Could you check a few things on this model? Use its own coordinates, in mm. Give positions to 0.01 mm unless a question says otherwise; leave off trailing zeros. Write each loop counter-clockwise with the first axis right and the second up, starting at its lowest first coordinate (ties: lowest second). Pieces come first, ordered by that corner, then holes. Notation, with made-up numbers: (16, 78) - (51, 78) arc R26 cw to (51, 101) - close; hole circle Ø1 at (30.25, 62.25). An arc over 180 degrees is marked (long way). Use one line per item in the form item = value.
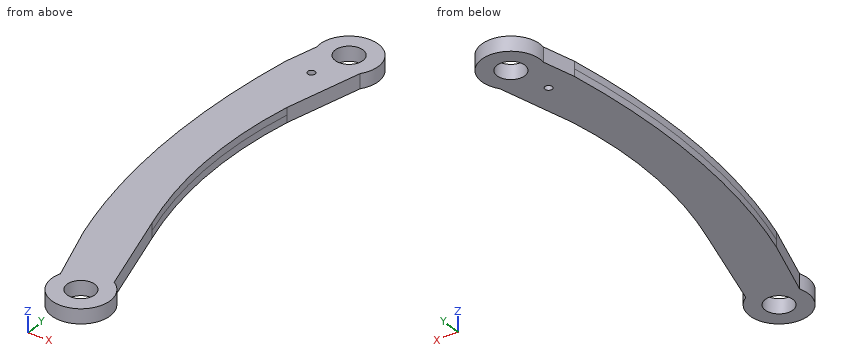
```python
from build123d import *

# Parameters (mm, degrees)
SKETCH1_R           = 1
SKETCH1_W           = 7.92
SKETCH1_H           = 7.92
SKETCH1_R_2         = 3.8
BOSS_EXTRUDE1_DEPTH = 2
SKETCH2_R           = 8
SKETCH2_W           = 7.92
SKETCH2_H           = 7.92
BOSS_EXTRUDE2_DEPTH = 2


with BuildPart() as part:
    # Sketch1 → Boss-Extrude1 (new body, symmetric)
    with BuildSketch(Plane.XY):
        with BuildLine():
            Line((-5.004193268, -11.768083729), (1.264827755, 12.086469882))
            ThreePointArc((1.264827755, 12.086469882), (-3.646245645, 20.982534185), (-12.767631248, 16.503814873))
            Line((-12.767631248, 16.503814873), (-16.10900409, 3.908669428))
            add(Edge.make_bspline(
                [(-16.10900409, 3.908669428), (-19.377716834, -15.242508961), (-20.646085271, -43.801923377), (-15.357286602, -71.564124193), (-13.027019985, -79.992281382)],
                knots=[0, 0, 0, 0, 0.615830564, 0.891753854, 0.891753854, 0.891753854, 0.891753854], degree=3))
            Line((-13.027019985, -79.992281382), (-5.967709179, -101.821397306))
            ThreePointArc((-5.967709179, -101.821397306), (-2.543292548, -94.302394888), (5.340555406, -96.773622937))
            Line((5.340555406, -96.773622937), (-2.58265982, -68.335822015))
            add(Edge.make_bspline(
                [(-2.58265982, -68.335822015), (-10.677441901, -40.31981723), (-5.004193268, -11.768083729)],
                knots=[0, 0, 0, 1, 1, 1], degree=2))
        make_face()
        with Locations((-8.672039016, 3.248347704)):
            Circle(SKETCH1_R, mode=Mode.SUBTRACT)
        with Locations((-5.857463234, 13.958219751)):
            Rectangle(SKETCH1_W, SKETCH1_H, mode=Mode.SUBTRACT)
        with BuildLine():
            ThreePointArc((6.239474416, -100), (6.010544893, -98.325368373), (5.340555406, -96.773622937))
            ThreePointArc((5.340555406, -96.773622937), (-2.543292548, -94.302394888), (-5.967709179, -101.821397306))
            ThreePointArc((-5.967709179, -101.821397306), (0.92078017, -106.171159119), (6.239474416, -100))
        make_face()
        with Locations((0, -100)):
            Rectangle(SKETCH1_W, SKETCH1_H, mode=Mode.SUBTRACT)
        with Locations((0, -100)):
            Rectangle(SKETCH1_W, SKETCH1_H)
        with Locations((0, -100)):
            Circle(SKETCH1_R_2, mode=Mode.SUBTRACT)
        with Locations((-5.857463234, 13.958219751)):
            Rectangle(SKETCH1_W, SKETCH1_H)
        with Locations((-5.857463234, 13.958219751)):
            Circle(SKETCH1_R_2, mode=Mode.SUBTRACT)
    extrude(amount=BOSS_EXTRUDE1_DEPTH, both=True)

    # Sketch2 → Boss-Extrude2 (add, symmetric)
    with BuildSketch(Plane.XY):
        with Locations((0, -100)):
            Circle(SKETCH2_R)
        with Locations((0, -100)):
            Rectangle(SKETCH2_W, SKETCH2_H, mode=Mode.SUBTRACT)
        with Locations((-5.857463234, 13.958219751)):
            Circle(SKETCH2_R)
        with Locations((-5.857463234, 13.958219751)):
            Rectangle(SKETCH2_W, SKETCH2_H, mode=Mode.SUBTRACT)
    extrude(amount=BOSS_EXTRUDE2_DEPTH, both=True)


solid = part.part
```
1. Imagine slicing it at A-A, the plane y = -100. List the corners of the cut face in (x, z) for me, and give its area (3 significant figures).
Response values:
outline = (-8, -2) - (-3.8, -2) - (-3.8, 2) - (-8, 2) - close; (3.8, -2) - (8, -2) - (8, 2) - (3.8, 2) - close
area = 33.6 mm²
2. If I drill on line 1 (X direction, y = -64, z = 1.8); line 2 (X direction, y = -47.5, z = -1.3); line 3 (Y direction, x = 6, z = -1), over which ranges is the centre line in solid material (lowest first)? Write a range as from..to.
Response values:
line_1 = -16.6..-3.75
line_2 = -18.67..-6.69
line_3 = -105.29..-94.71
3. For pin 1 (1 mm diameter, centred on y = -71, z = 0, fed in from +X); pin 2 (2 mm diameter, centred on x = -9.5, z = -1, fed in from +Y); pin 3 (1.8 mm diameter, centred on x = -8.67, y = 3.25, fed in from -Z), each with a flat end and sliding along its axis, tell me the tip position at first contact or that it passes through.
Response values:
pin_1 = -1.7
pin_2 = 21.51
pin_3 = through
4. Imagine slicing it at B-B, the plane z = -1.1. State how many separate pieces and enclosed holes the cut face has, and give its area (3 significant figures).
Response values:
separate_pieces = 1
enclosed_holes = 3
area = 1,620 mm²
